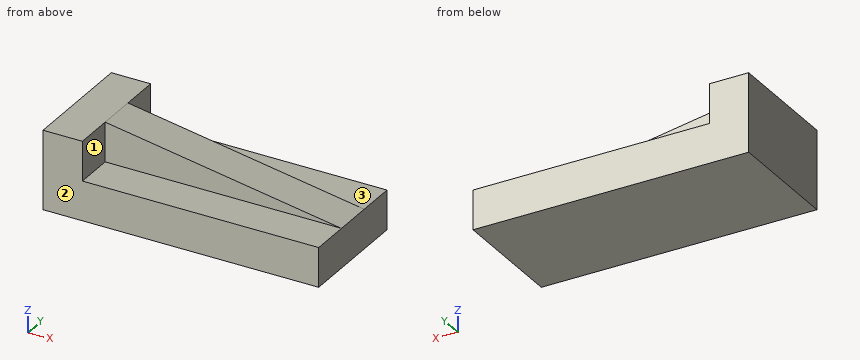
```python
from build123d import *

# Parameters (mm, degrees)
F1_DEPTH = 76.2
F3_DEPTH = 25.4
F5_DEPTH = 25.4


with BuildPart() as f1:
    # F0 (on Front) → F1 (new body)
    with BuildSketch(Plane.XZ):
        Polygon((0, 50.8), (0, 0), (177.8, 0), (177.8, 25.4), (25.4, 25.4), (25.4, 50.8), align=None)
        Polygon((177.8, 25.4), (25.4, 50.8), (25.4, 25.4), align=None)
    extrude(amount=-F1_DEPTH)

    # F2 (on face) → F3 (cut)
    with BuildSketch(Plane.XZ):
        Polygon((177.8, 25.4), (25.4, 50.8), (25.4, 25.4), align=None)
    extrude(amount=-F3_DEPTH, mode=Mode.SUBTRACT)

    # F4 (on face) → F5 (cut)
    with BuildSketch(Plane(origin=(0, 76.2, 0), x_dir=(-1, 0, 0), z_dir=(0, 1, 0))):
        Polygon((-25.4, 25.4), (-25.4, 50.8), (-177.8, 25.4), align=None)
    extrude(amount=-F5_DEPTH, mode=Mode.SUBTRACT)


solid = f1.part
```
Geometry check sheet. Reference: the model listing, model coordinates, mm. Face numbers are marked on the shaded views. A direction names the side the tool comes from. Give positions to 0.01 mm unless a question says otherwise; leave off trailing zeros. Loops run counter-clockwise (first coordinate to the right, second up) from the corner with the lowest first, then second, coordinate; pieces in that order, holes last. Notation, with made-up numbers: M 62.5,1 L 88.5,1 A11 ccw 88.5,14 Z; hole C 21,76.5 d9. An arc over 180 degrees is marked long. Write item = value, one per line. Start each with the question number.
1. Section check A-A, the plane x = 116. Enter the section's corners in (y, z).
2. Go/stop test with flat-tipped pins: P1, Ø20.5, axis at x = 66, y = 60, coming from the +Z side; P2, Ø7.5, axis at y = 68, z = 37.5, coming from the +X side; P3, Ø8, axis at x = 107.5, z = 31, coming from the -Y side. Record where each tip stops, or that it passes through.
3. Thickness scan on probe 1 along Z at (x, y) = (161.5, 19); probe 2 along Y at (x, z) = (103.5, 28). Record the ranges inside material, lowest first.
4. Section check D-D, the plane y = 56. Enter the section's corners in (x, z), plus the area to 3 significant figures.
5. Tool access check on the marked faces 1, 2 and 3. Record the directions out of +Z, -Z, +X, -X, +Y, -Y that give a thin tool (end or side, any length) a straight path to the whole face; none if there is none.
6. Section check C-C, the plane y = 46.5. Enter the section's corners in (x, z), plus the area to 3 significant figures.
7. Section check B-B, the plane z = 32. Enter the section's corners in (x, y).
Values follow:
q1.outline = M 0,0 L 76.2,0 L 76.2,25.4 L 50.8,25.4 L 50.8,35.7 L 25.4,35.7 L 25.4,25.4 L 0,25.4 Z
q2.P1 = 44.79
q2.P2 = 25.4
q2.P3 = 25.4
q3.probe_1 = 0 to 25.4
q3.probe_2 = 25.4 to 50.8
q4.outline = M 0,0 L 177.8,0 L 177.8,25.4 L 25.4,25.4 L 25.4,50.8 L 0,50.8 Z
q4.area = 5,160 mm^2
q5.face_1 = +Z, +X, -Y
q5.face_2 = +Z, -Z, +X, -X, -Y
q5.face_3 = +Z, +X, +Y
q6.outline = M 0,0 L 177.8,0 L 177.8,25.4 L 25.4,50.8 L 0,50.8 Z
q6.area = 7,100 mm^2
q7.outline = M 0,0 L 25.4,0 L 25.4,25.4 L 138.2,25.4 L 138.2,50.8 L 25.4,50.8 L 25.4,76.2 L 0,76.2 Z
